from build123d import *

# Parameters (mm, degrees)
SKETCH2_W                = 5
SKETCH2_H                = 5
BOSS_EXTRUDE1_DEPTH      = 2.5
BOSS_EXTRUDE2_DEPTH      = 5
BOSS_EXTRUDE3_DEPTH      = 5
SKETCH5_W                = 0.5
SKETCH5_H                = 5
BOSS_EXTRUDE4_DEPTH      = 1
SKETCH6_W                = 5
SKETCH6_H                = 0.5
BOSS_EXTRUDE5_DEPTH      = 1
MIRROR3_START            = -2.5
MIRROR3_OUTLINE_W        = 0.5
MIRROR3_OUTLINE_H        = 1
MIRROR3_DEPTH            = 5
MIRROR5_COPY_1_DEPTH     = 5
MIRROR5_COPY_2_DEPTH     = 5
MIRROR6_START            = -2.5
MIRROR6_OUTLINE_W        = 1
MIRROR6_OUTLINE_H        = 0.5
MIRROR6_DEPTH            = 5
BOSS_EXTRUDE7_DEPTH      = 5
BOSS_EXTRUDE9_DEPTH      = 5
SKETCH10_W               = 5
SKETCH10_H               = 1
CUT_EXTRUDE1_DEPTH       = 12.543396381
SKETCH11_W               = 5
SKETCH11_H               = 5
BOSS_EXTRUDE11_DEPTH     = 1.5
BOSS_EXTRUDE13_DEPTH     = 5
BOSS_EXTRUDE14_DEPTH     = 5
SKETCH15_W               = 0.5
SKETCH15_H               = 5
BOSS_EXTRUDE15_DEPTH     = 0.75
SKETCH16_W               = 5
SKETCH16_H               = 0.5
BOSS_EXTRUDE16_DEPTH     = 0.75
MIRROR16_COPY_1_SKETCH_W = 0.5
MIRROR16_COPY_1_SKETCH_H = 5
MIRROR16_COPY_1_DEPTH    = 0.75
MIRROR16_COPY_2_SKETCH_W = 5
MIRROR16_COPY_2_SKETCH_H = 0.5
MIRROR16_COPY_2_DEPTH    = 0.75
MIRROR18_COPY_1_DEPTH    = 5
BOSS_EXTRUDE18_DEPTH     = 5
BOSS_EXTRUDE19_DEPTH     = 5
SKETCH20_W               = 5
SKETCH20_H               = 5
BOSS_EXTRUDE20_DEPTH     = 1.5
BOSS_EXTRUDE21_DEPTH     = 5
BOSS_EXTRUDE22_DEPTH     = 5
SKETCH23_W               = 0.4
SKETCH23_H               = 5
BOSS_EXTRUDE23_DEPTH     = 0.5
SKETCH24_W               = 5
SKETCH24_H               = 0.4
BOSS_EXTRUDE24_DEPTH     = 0.5
MIRROR24_START           = -2.5
MIRROR24_OUTLINE_W       = 0.4
MIRROR24_OUTLINE_H       = 0.5
MIRROR24_DEPTH           = 5
MIRROR25_START           = -2.5
MIRROR25_DEPTH           = 5
MIRROR26_START           = -2.5
MIRROR26_OUTLINE_W       = 0.5
MIRROR26_OUTLINE_H       = 0.4
MIRROR26_DEPTH           = 5
BOSS_EXTRUDE25_DEPTH     = 5
BOSS_EXTRUDE26_DEPTH     = 5
SKETCH27_W               = 9
SKETCH27_H               = 9
BOSS_EXTRUDE27_DEPTH     = 1.5


# Read off the part's stored shape, not the designer's step: Mirror3, Mirror6, Mirror24, Mirror25, Mirror26
with BuildPart() as part:
    # Sketch2 → Boss-Extrude1 (new body)
    with BuildSketch(Plane(origin=(0, 0, 0), x_dir=(1, 0, 0), z_dir=(0, 1, 0))):
        Rectangle(SKETCH2_W, SKETCH2_H)
    boss_extrude1 = extrude(amount=BOSS_EXTRUDE1_DEPTH)

    # Sketch3 → Boss-Extrude2 (add)
    with BuildSketch(Plane.XY.offset(2.5)):
        Polygon((-2.5, 1.5), (-4, 3), (-4.5, 3), (-2.5, 1), align=None)
    boss_extrude2 = extrude(amount=-BOSS_EXTRUDE2_DEPTH)

    # Sketch4 → Boss-Extrude3 (add)
    with BuildSketch(Plane(origin=(2.5, 0, 0), x_dir=(0, 0, -1), z_dir=(1, 0, 0))):
        Polygon((2.5, 1.5), (2.5, 1), (4.5, 3), (4, 3), align=None)
    boss_extrude3 = extrude(amount=-BOSS_EXTRUDE3_DEPTH)

    # Sketch5 → Boss-Extrude4 (add)
    with BuildSketch(Plane(origin=(0, 3, 0), x_dir=(1, 0, 0), z_dir=(0, 1, 0))):
        with Locations((-4.25, 0)):
            Rectangle(SKETCH5_W, SKETCH5_H)
    boss_extrude4 = extrude(amount=BOSS_EXTRUDE4_DEPTH)

    # Sketch6 → Boss-Extrude5 (add)
    with BuildSketch(Plane(origin=(0, 3, 0), x_dir=(1, 0, 0), z_dir=(0, 1, 0))):
        with Locations((0, 4.25)):
            Rectangle(SKETCH6_W, SKETCH6_H)
    boss_extrude5 = extrude(amount=BOSS_EXTRUDE5_DEPTH)

    # Mirror1: Boss-Extrude3, Boss-Extrude5 across plane
    add(boss_extrude3.mirror(Plane.XY))
    add(boss_extrude5.mirror(Plane.XY))

    # Mirror2: Boss-Extrude2, Boss-Extrude4 across plane
    add(boss_extrude2.mirror(Plane(origin=(0, 0, 0), x_dir=(0, 0, 1), z_dir=(1, 0, 0))))
    add(boss_extrude4.mirror(Plane(origin=(0, 0, 0), x_dir=(0, 0, 1), z_dir=(1, 0, 0))))

    # Mirror3 outline → Mirror3 (add)
    with BuildSketch(Plane.XY.offset(MIRROR3_START)):
        with Locations((-4.25, 4.5)):
            Rectangle(MIRROR3_OUTLINE_W, MIRROR3_OUTLINE_H)
        with Locations((4.25, 4.5)):
            Rectangle(MIRROR3_OUTLINE_W, MIRROR3_OUTLINE_H)
    extrude(amount=MIRROR3_DEPTH)

    # Mirror4: Boss-Extrude2 across plane
    add(boss_extrude2.mirror(Plane.ZX.offset(4)))

    # Mirror5 copy 1 sketch → Mirror5 copy 1 (add)
    with BuildSketch(Plane(origin=(0, 8, 2.5), x_dir=(-1, 0, 0), z_dir=(0, 0, 1))):
        Polygon((-2.5, 1.5), (-4, 3), (-4.5, 3), (-2.5, 1), align=None)
    extrude(amount=-MIRROR5_COPY_1_DEPTH)

    # Mirror5 copy 2 sketch → Mirror5 copy 2 (add)
    with BuildSketch(Plane(origin=(0, 0, 2.5), x_dir=(-1, 0, 0), z_dir=(0, 0, 1))):
        Polygon((-2.5, -1.5), (-4, -3), (-4.5, -3), (-2.5, -1), align=None)
    extrude(amount=-MIRROR5_COPY_2_DEPTH)

    # Mirror6 outline → Mirror6 (add)
    with BuildSketch(Plane.YZ.offset(MIRROR6_START)):
        with Locations((4.5, -4.25)):
            Rectangle(MIRROR6_OUTLINE_W, MIRROR6_OUTLINE_H)
        with Locations((4.5, 4.25)):
            Rectangle(MIRROR6_OUTLINE_W, MIRROR6_OUTLINE_H)
    extrude(amount=MIRROR6_DEPTH)

    # Mirror10: Boss-Extrude1 across plane
    add(boss_extrude1.mirror(Plane.ZX.offset(4)))

    # Sketch10 → Cut-Extrude1 (cut, through all)
    with BuildSketch(Plane.XY.offset(2.5)):
        with Locations((0, 7.5)):
            Rectangle(SKETCH10_W, SKETCH10_H)
    extrude(amount=-CUT_EXTRUDE1_DEPTH, mode=Mode.SUBTRACT)



with BuildPart() as body_2:
    # Sketch7 → Boss-Extrude7 (new body)
    with BuildSketch(Plane.ZY.offset(2.5)):
        Polygon((-4.5, 5), (-4, 5), (-2.5, 6.5), (-2.5, 7), align=None)
    extrude(amount=-BOSS_EXTRUDE7_DEPTH)


with BuildPart() as body_3:
    # Sketch8 → Boss-Extrude9 (new body)
    with BuildSketch(Plane.ZY.offset(2.5)):
        Polygon((4.5, 5), (4, 5), (2.5, 6.5), (2.5, 7), align=None)
    extrude(amount=-BOSS_EXTRUDE9_DEPTH)


with BuildPart() as part_1:
    add(part.part)

    add(body_2.part)  # Boss-Extrude11 merges body 2

    add(body_3.part)  # Boss-Extrude11 merges body 3
    # Sketch11 → Boss-Extrude11 (add)
    with BuildSketch(Plane(origin=(0, 7, 0), x_dir=(1, 0, 0), z_dir=(0, 1, 0))):
        Rectangle(SKETCH11_W, SKETCH11_H)
    boss_extrude11 = extrude(amount=BOSS_EXTRUDE11_DEPTH)

    # Sketch13 → Boss-Extrude13 (add)
    with BuildSketch(Plane.ZY.offset(2.5)):
        Polygon((2.5, 7), (2.5, 7.5), (4, 9), (4.5, 9), align=None)
    boss_extrude13 = extrude(amount=-BOSS_EXTRUDE13_DEPTH)

    # Sketch14 → Boss-Extrude14 (add)
    with BuildSketch(Plane(origin=(0, 0, -2.5), x_dir=(-1, 0, 0), z_dir=(0, 0, -1))):
        Polygon((2.5, 7), (4.5, 9), (4, 9), (2.5, 7.5), align=None)
    boss_extrude14 = extrude(amount=-BOSS_EXTRUDE14_DEPTH)

    # Mirror12: Boss-Extrude13 across plane
    add(boss_extrude13.mirror(Plane.XY))

    # Mirror13: Boss-Extrude14 across plane
    add(boss_extrude14.mirror(Plane(origin=(0, 0, 0), x_dir=(0, 0, 1), z_dir=(1, 0, 0))))

    # Sketch15 → Boss-Extrude15 (add)
    with BuildSketch(Plane(origin=(0, 9, 0), x_dir=(1, 0, 0), z_dir=(0, 1, 0))):
        with Locations((-4.25, 0)):
            Rectangle(SKETCH15_W, SKETCH15_H)
    boss_extrude15 = extrude(amount=BOSS_EXTRUDE15_DEPTH)

    # Sketch16 → Boss-Extrude16 (add)
    with BuildSketch(Plane(origin=(0, 9, 0), x_dir=(1, 0, 0), z_dir=(0, 1, 0))):
        with Locations((0, 4.25)):
            Rectangle(SKETCH16_W, SKETCH16_H)
    boss_extrude16 = extrude(amount=BOSS_EXTRUDE16_DEPTH)

    # Mirror14: Boss-Extrude15 across plane
    add(boss_extrude15.mirror(Plane(origin=(0, 0, 0), x_dir=(0, 0, 1), z_dir=(1, 0, 0))))

    # Mirror15: Boss-Extrude16 across plane
    add(boss_extrude16.mirror(Plane.XY))

    # Mirror16: Boss-Extrude15, Boss-Extrude16 across plane
    add(boss_extrude15.mirror(Plane.ZX.offset(9.75)))
    add(boss_extrude16.mirror(Plane.ZX.offset(9.75)))

    # Mirror16 copy 1 sketch → Mirror16 copy 1 (add)
    with BuildSketch(Plane(origin=(0, 10.5, 0), x_dir=(-1, 0, 0), z_dir=(0, -1, 0))):
        with Locations((-4.25, 0)):
            Rectangle(MIRROR16_COPY_1_SKETCH_W, MIRROR16_COPY_1_SKETCH_H)
    extrude(amount=MIRROR16_COPY_1_DEPTH)

    # Mirror16 copy 2 sketch → Mirror16 copy 2 (add)
    with BuildSketch(Plane.XZ.offset(-10.5)):
        with Locations((0, 4.25)):
            Rectangle(MIRROR16_COPY_2_SKETCH_W, MIRROR16_COPY_2_SKETCH_H)
    extrude(amount=MIRROR16_COPY_2_DEPTH)

    # Mirror18: Boss-Extrude14 across plane
    add(boss_extrude14.mirror(Plane.ZX.offset(9.75)))

    # Mirror18 copy 1 sketch → Mirror18 copy 1 (add)
    with BuildSketch(Plane(origin=(0, 19.5, -2.5), x_dir=(1, 0, 0), z_dir=(0, 0, -1))):
        Polygon((2.5, 7), (4.5, 9), (4, 9), (2.5, 7.5), align=None)
    extrude(amount=-MIRROR18_COPY_1_DEPTH)

    # Mirror21: Boss-Extrude11 across plane
    add(boss_extrude11.mirror(Plane.ZX.offset(9.75)))



with BuildPart() as body_2_2:
    # Sketch17 → Boss-Extrude18 (new body)
    with BuildSketch(Plane(origin=(2.5, 0, 0), x_dir=(0, 0, -1), z_dir=(1, 0, 0))):
        Polygon((4, 10.5), (4.5, 10.5), (2.5, 12.5), (2.5, 12), align=None)
    extrude(amount=-BOSS_EXTRUDE18_DEPTH)


with BuildPart() as body_3_2:
    # Sketch18 → Boss-Extrude19 (new body)
    with BuildSketch(Plane(origin=(2.5, 0, 0), x_dir=(0, 0, -1), z_dir=(1, 0, 0))):
        Polygon((-4.5, 10.5), (-4, 10.5), (-2.5, 12), (-2.5, 12.5), align=None)
    extrude(amount=-BOSS_EXTRUDE19_DEPTH)


with BuildPart() as part_2:
    add(part_1.part)

    add(body_2_2.part)  # Boss-Extrude20 merges body 2 2

    add(body_3_2.part)  # Boss-Extrude20 merges body 3 2
    # Sketch20 → Boss-Extrude20 (add)
    with BuildSketch(Plane(origin=(0, 12.5, 0), x_dir=(1, 0, 0), z_dir=(0, 1, 0))):
        Rectangle(SKETCH20_W, SKETCH20_H)
    boss_extrude20 = extrude(amount=BOSS_EXTRUDE20_DEPTH)

    # Sketch21 → Boss-Extrude21 (add)
    with BuildSketch(Plane.XY.offset(2.5)):
        Polygon((2.5, 12.5), (2.5, 12.9), (4.1, 14.5), (4.5, 14.5), align=None)
    boss_extrude21 = extrude(amount=-BOSS_EXTRUDE21_DEPTH)

    # Sketch22 → Boss-Extrude22 (add)
    with BuildSketch(Plane.ZY.offset(2.5)):
        Polygon((2.5, 12.5), (2.5, 12.9), (4.1, 14.5), (4.5, 14.5), align=None)
    boss_extrude22 = extrude(amount=-BOSS_EXTRUDE22_DEPTH)

    # Sketch23 → Boss-Extrude23 (add)
    with BuildSketch(Plane(origin=(0, 14.5, 0), x_dir=(1, 0, 0), z_dir=(0, 1, 0))):
        with Locations((4.3, 0)):
            Rectangle(SKETCH23_W, SKETCH23_H)
    boss_extrude23 = extrude(amount=BOSS_EXTRUDE23_DEPTH)

    # Sketch24 → Boss-Extrude24 (add)
    with BuildSketch(Plane(origin=(0, 14.5, 0), x_dir=(1, 0, 0), z_dir=(0, 1, 0))):
        with Locations((0, -4.3)):
            Rectangle(SKETCH24_W, SKETCH24_H)
    boss_extrude24 = extrude(amount=BOSS_EXTRUDE24_DEPTH)

    # Mirror22: Boss-Extrude22, Boss-Extrude24 across plane
    add(boss_extrude22.mirror(Plane.XY))
    add(boss_extrude24.mirror(Plane.XY))

    # Mirror23: Boss-Extrude21, Boss-Extrude23 across plane
    add(boss_extrude21.mirror(Plane(origin=(0, 0, 0), x_dir=(0, 0, 1), z_dir=(1, 0, 0))))
    add(boss_extrude23.mirror(Plane(origin=(0, 0, 0), x_dir=(0, 0, 1), z_dir=(1, 0, 0))))

    # Mirror24 outline → Mirror24 (add)
    with BuildSketch(Plane.XY.offset(MIRROR24_START)):
        with Locations((-4.3, 15.25)):
            Rectangle(MIRROR24_OUTLINE_W, MIRROR24_OUTLINE_H)
        with Locations((4.3, 15.25)):
            Rectangle(MIRROR24_OUTLINE_W, MIRROR24_OUTLINE_H)
    extrude(amount=MIRROR24_DEPTH)

    # Mirror25 outline → Mirror25 (add)
    with BuildSketch(Plane.XY.offset(MIRROR25_START)):
        Polygon((-2.5, 17.1), (-2.5, 17.5), (-4.5, 15.5), (-4.1, 15.5), align=None)
        Polygon((4.5, 15.5), (2.5, 17.5), (2.5, 17.1), (4.1, 15.5), align=None)
    extrude(amount=MIRROR25_DEPTH)

    # Mirror26 outline → Mirror26 (add)
    with BuildSketch(Plane.YZ.offset(MIRROR26_START)):
        with Locations((15.25, -4.3)):
            Rectangle(MIRROR26_OUTLINE_W, MIRROR26_OUTLINE_H)
        with Locations((15.25, 4.3)):
            Rectangle(MIRROR26_OUTLINE_W, MIRROR26_OUTLINE_H)
    extrude(amount=MIRROR26_DEPTH)

    # Mirror28: Boss-Extrude20 across plane
    add(boss_extrude20.mirror(Plane.ZX.offset(15)))



with BuildPart() as body_2_3:
    # Sketch25 → Boss-Extrude25 (new body)
    with BuildSketch(Plane.ZY.offset(2.5)):
        Polygon((4.1, 15.5), (4.5, 15.5), (2.5, 17.5), (2.5, 17.1), align=None)
    extrude(amount=-BOSS_EXTRUDE25_DEPTH)


with BuildPart() as body_3_3:
    # Sketch26 → Boss-Extrude26 (new body)
    with BuildSketch(Plane.ZY.offset(2.5)):
        Polygon((-4.1, 15.5), (-4.5, 15.5), (-2.5, 17.5), (-2.5, 17.1), align=None)
    extrude(amount=-BOSS_EXTRUDE26_DEPTH)


with BuildPart() as part_3:
    add(part_2.part)

    add(body_2_3.part)  # Boss-Extrude27 merges body 2 3

    add(body_3_3.part)  # Boss-Extrude27 merges body 3 3
    # Sketch27 → Boss-Extrude27 (add)
    with BuildSketch(Plane(origin=(0, 17.5, 0), x_dir=(1, 0, 0), z_dir=(0, 1, 0))):
        Rectangle(SKETCH27_W, SKETCH27_H)
    extrude(amount=BOSS_EXTRUDE27_DEPTH)


solid = part_3.part
For this review, take the finished solid that the model builds, in its own axes (mm). A direction names the side the tool comes from. Give positions to 0.01 mm unless a question says otherwise; leave off trailing zeros. Loops run counter-clockwise (first coordinate to the right, second up) from the corner with the lowest first, then second, coordinate; pieces in that order, holes last. Notation, with made-up numbers: M 44,78.5 L 100,78.5 A14 ccw 100,85.5 Z; hole C 7,57 d9. An arc over 180 degrees is marked long. Answer as a JSON object with one key per item and string values. Group by question number.
Q1. Mouldability with a two-part tool opening along Z and no side actions: class faces 1 (the flat face through (0, 2.5, 0)), 2 (the flat face through (3.3, 11.2, 0)), 3 (the flat face through (0, 0.5, -2.5)), 4 (the flat face through (0, 14, 0)) as +Z half, -Z half, draft (parallel to the pull), parting line (faces both ways), or undercut.
Q2. Insertion check: P1, Ø1.6, axis at y = 4, z = -3.5, coming from the +X side; P2, Ø1.1, axis at y = 2, z = -0.5, coming from the -X side; P3, Ø0.9, axis at x = 1, y = 13, coming from the -Z side. Each pin has a flat end and moves straight along its axis. Give the tip position at first contact, or say it passes through.
Q3. For probe 1 along Y at (x, z) = (1, 1.5); probe 2 along X at (y, z) = (11.25, -1); probe 3 along Z at (x, y) = (-0.25, 11.5), list the stretches that pass through material, from the lowest coordinate up. Write a range as [from, to].
Q4. Add section A-A on x = 3. Give the boundary of the cut face in (y, z), and give its area (3 significant figures).
Q5. Add section C-C on z = 3. Give the boundary of the cut face in (x, y).
Q6. Add section B-B on y = 15. Give the boundary of the cut face in (x, z), and give its area (3 significant figures).
Q7. Tool access review of faces 5 (the flat face through (3.5, 8, 0)), 6 (the flat face through (0, 14, 4)), 7 (the flat face through (0, 16.3, 3.3)), 8 (the flat face through (3, 2, 0)), 9 (the flat face through (-2.5, 9.8, -4.2)): name each direction out of +Z, -Z, +X, -X, +Y, -Y from which nothing blocks a thin tool from reaching the whole face with its end or side.
Q8. Add section D-D on y = 6.25. Give the boundary of the cut face in (x, z), and give its area (3 significant figures).
Checked values:
{
 "1": {"face 1": "undercut", "face 2": "draft", "face 3": "-Z half", "face 4": "undercut"},
 "2": {"P1": "x = 2.5", "P2": "x = -4.05", "P3": "z = -3.45"},
 "3": {"probe 1": "[0, 2.5], [5.5, 8.5], [11, 14], [16, 19]", "probe 2": "[-3.75, -3.25], [-2.5, 2.5], [3.25, 3.75]", "probe 3": "[-3.5, -3], [-2.5, 2.5], [3, 3.5]"},
 "4": {"outline": "M 1.5,-2.5 L 2,-2.5 L 2,2.5 L 1.5,2.5 Z; M 6,-2.5 L 6.5,-2.5 L 6.5,2.5 L 6,2.5 Z; M 7.5,-2.5 L 8,-2.5 L 8,2.5 L 7.5,2.5 Z; M 11.5,-2.5 L 12,-2.5 L 12,2.5 L 11.5,2.5 Z; M 13,-2.5 L 13.4,-2.5 L 13.4,2.5 L 13,2.5 Z; M 16.6,-2.5 L 17,-2.5 L 17,2.5 L 16.6,2.5 Z; M 17.5,-4.5 L 19,-4.5 L 19,4.5 L 17.5,4.5 Z", "area": "27.5 mm²"},
 "5": {"outline": "M -4.5,17.5 L 4.5,17.5 L 4.5,19 L -4.5,19 Z; M -2.5,1.5 L 2.5,1.5 L 2.5,2 L -2.5,2 Z; M -2.5,6 L 2.5,6 L 2.5,6.5 L -2.5,6.5 Z; M -2.5,7.5 L 2.5,7.5 L 2.5,8 L -2.5,8 Z; M -2.5,11.5 L 2.5,11.5 L 2.5,12 L -2.5,12 Z; M -2.5,13 L 2.5,13 L 2.5,13.4 L -2.5,13.4 Z; M -2.5,16.6 L 2.5,16.6 L 2.5,17 L -2.5,17 Z"},
 "6": {"outline": "M -4.5,-2.5 L -4.1,-2.5 L -4.1,2.5 L -4.5,2.5 Z; M -2.5,-4.5 L 2.5,-4.5 L 2.5,-4.1 L -2.5,-4.1 Z; M -2.5,4.1 L 2.5,4.1 L 2.5,4.5 L -2.5,4.5 Z; M 4.1,-2.5 L 4.5,-2.5 L 4.5,2.5 L 4.1,2.5 Z", "area": "8.00 mm²"},
 "7": {"face 5": "+Z, -Z, +X", "face 6": "+Z, +X, -X", "face 7": "+X, -X", "face 8": "+Z, -Z", "face 9": "-Z, -X, -Y"},
 "8": {"outline": "M -3.25,-2.5 L -2.75,-2.5 L -2.75,2.5 L -3.25,2.5 Z; M -2.5,-3.25 L 2.5,-3.25 L 2.5,-2.75 L -2.5,-2.75 Z; M -2.5,-2.5 L 2.5,-2.5 L 2.5,2.5 L -2.5,2.5 Z; M -2.5,2.75 L 2.5,2.75 L 2.5,3.25 L -2.5,3.25 Z; M 2.75,-2.5 L 3.25,-2.5 L 3.25,2.5 L 2.75,2.5 Z", "area": "35.0 mm²"}
}
